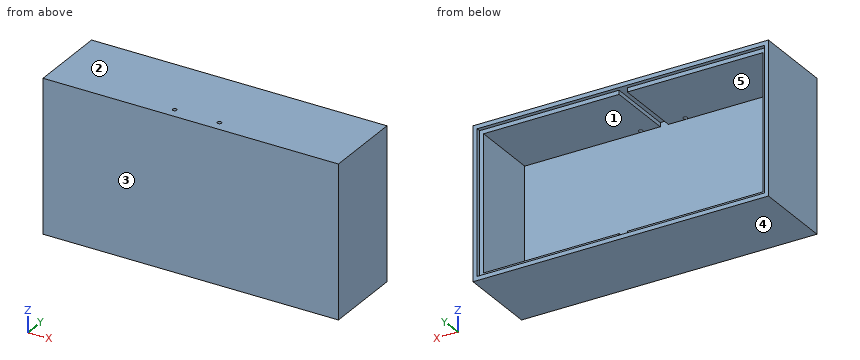
from build123d import *

# Parameters (mm, degrees)
SKETCH1_W           = 109
SKETCH1_H           = 112
BOSS_EXTRUDE1_DEPTH = 59
SKETCH2_W           = 97
SKETCH2_H           = 100
SKETCH2_W_2         = 3
SKETCH2_H_2         = 50
CUT_EXTRUDE1_DEPTH  = 53
SKETCH2_3_W         = 103
SKETCH2_3_H         = 106
SKETCH2_3_W_2       = 97
SKETCH2_3_H_2       = 100
CUT_EXTRUDE2_DEPTH  = 3
SKETCH6_R           = 1.5
CUT_EXTRUDE28_DEPTH = 6


with BuildPart() as part:
    # Sketch1 → Boss-Extrude1 (new body)
    with BuildSketch(Plane(origin=(0, 0, 0), x_dir=(1, 0, 0), z_dir=(0, 1, 0))):
        with Locations((-54.5, 0)):
            Rectangle(SKETCH1_W, SKETCH1_H)
    boss_extrude1 = extrude(amount=BOSS_EXTRUDE1_DEPTH)

    # Sketch2 → Cut-Extrude1 (cut)
    with BuildSketch(Plane(origin=(0, 59, 0), x_dir=(1, 0, 0), z_dir=(0, 1, 0))):
        with Locations((-54.5, 0)):
            Rectangle(SKETCH2_W, SKETCH2_H)
        Polygon((0, 0), (-3, 0), (-3, -50), (-3, -53), (0, -53), align=None)
        Polygon((-3, 53), (-3, 50), (-3, 0), (0, 0), (0, 53), align=None)
        with Locations((-4.5, -25)):
            Rectangle(SKETCH2_W_2, SKETCH2_H_2)
        with Locations((-4.5, 25)):
            Rectangle(SKETCH2_W_2, SKETCH2_H_2)
    cut_extrude1 = extrude(amount=-CUT_EXTRUDE1_DEPTH, mode=Mode.SUBTRACT)

    # Sketch2_3 → Cut-Extrude2 (cut)
    with BuildSketch(Plane(origin=(0, 59, 0), x_dir=(1, 0, 0), z_dir=(0, 1, 0))):
        with Locations((-54.5, 0)):
            Rectangle(SKETCH2_3_W, SKETCH2_3_H)
        with Locations((-54.5, 0)):
            Rectangle(SKETCH2_3_W_2, SKETCH2_3_H_2, mode=Mode.SUBTRACT)
    cut_extrude2 = extrude(amount=-CUT_EXTRUDE2_DEPTH, mode=Mode.SUBTRACT)

    # Sketch6 → Cut-Extrude28 (cut)
    with BuildSketch(Plane.XY.offset(56)):
        with Locations((-16.5, 7.7)):
            Circle(SKETCH6_R)
    cut_extrude28 = extrude(amount=-CUT_EXTRUDE28_DEPTH, mode=Mode.SUBTRACT)

    # Mirror1: Boss-Extrude1, Cut-Extrude1, Cut-Extrude2, Cut-Extrude28 across plane
    add(boss_extrude1.mirror(Plane(origin=(0, 0, 0), x_dir=(0, 0, 1), z_dir=(1, 0, 0))))
    add(cut_extrude1.mirror(Plane(origin=(0, 0, 0), x_dir=(0, 0, 1), z_dir=(1, 0, 0))), mode=Mode.SUBTRACT)
    add(cut_extrude2.mirror(Plane(origin=(0, 0, 0), x_dir=(0, 0, 1), z_dir=(1, 0, 0))), mode=Mode.SUBTRACT)
    add(cut_extrude28.mirror(Plane(origin=(0, 0, 0), x_dir=(0, 0, 1), z_dir=(1, 0, 0))), mode=Mode.SUBTRACT)


solid = part.part
Part model, mm, in its own coordinate system. Face numbers are marked on the shaded views. A direction names the side the tool comes from. Coordinates: 2 decimals unless noted, no trailing zeros. Order: outer loops, then holes, each group sorted by start corner. A loop starts at its lowest first (then second) coordinate and runs counter-clockwise, first axis right, second up. Notation, with made-up numbers: M 44,63.5 L 67,63.5 A24 cw 67,85.5 Z; hole C 17.5,62 d5. An arc over 180 degrees is marked long. One line per question, with ' | ' between items.
Q1. Slice it at A-A (y = 38.5). Give the cut face in (x, z).
A:
outline: M -109,-56 L 109,-56 L 109,56 L -109,56 Z; hole M -103,-50 L -3,-50 L -3,-53 L 3,-53 L 3,-50 L 103,-50 L 103,50 L 3,50 L 3,53 L -3,53 L -3,50 L -103,50 Z
Q2. Pin check, flat tips, straight feed: P1, Ø10, axis at x = 23, z = -8.5, coming from the -Y side; P2, Ø3, axis at x = -66, z = 6.5, coming from the +Y side. Stop position of each tip, or through.
A:
P1: stops at y = 0 | P2: stops at y = 6
Q3. Slice it at C-C (z = -7). Give the cut face in (x, y), and give its area (3 significant figures).
A:
outline: M -109,0 L 109,0 L 109,59 L 106,59 L 106,56 L 103,56 L 103,6 L -103,6 L -103,56 L -106,56 L -106,59 L -109,59 Z | area: 1,930 mm^2
Q4. Two-plate mould, pull along Z, no slides. Class the marked faces 1, 2 and 3: +Z half, -Z half, draft (parallel to the pull), parting line (faces both ways), or undercut.
A:
face 1: undercut | face 2: +Z half | face 3: draft
Q5. Slice it at B-B (x = 78). Give the cut face in (y, z).
A:
outline: M 0,-56 L 59,-56 L 59,-53 L 56,-53 L 56,-50 L 6,-50 L 6,50 L 56,50 L 56,53 L 59,53 L 59,56 L 0,56 Z
Q6. Drill centre lines: line 1 (X direction, y = 52, z = 6); line 2 (Y direction, x = -16.5, z = 53.4); line 3 (Z direction, x = 96, y = 57). Where is each one in solid material? Low to high.
A:
line 1: x = -109 to -103, 103 to 109 | line 2: y = 0 to 6.2, 9.2 to 59 | line 3: z = -56 to -53, 53 to 56
Q7. 3-axis set-ups, long thin cutter, end or side, ignore diameter. For the marked faces 4 and 5: which of +Z, -Z, +X, -X, +Y, -Y reach the whole face in a straight line?
A:
face 4: -Z, +X, -X, +Y, -Y | face 5: +Y
